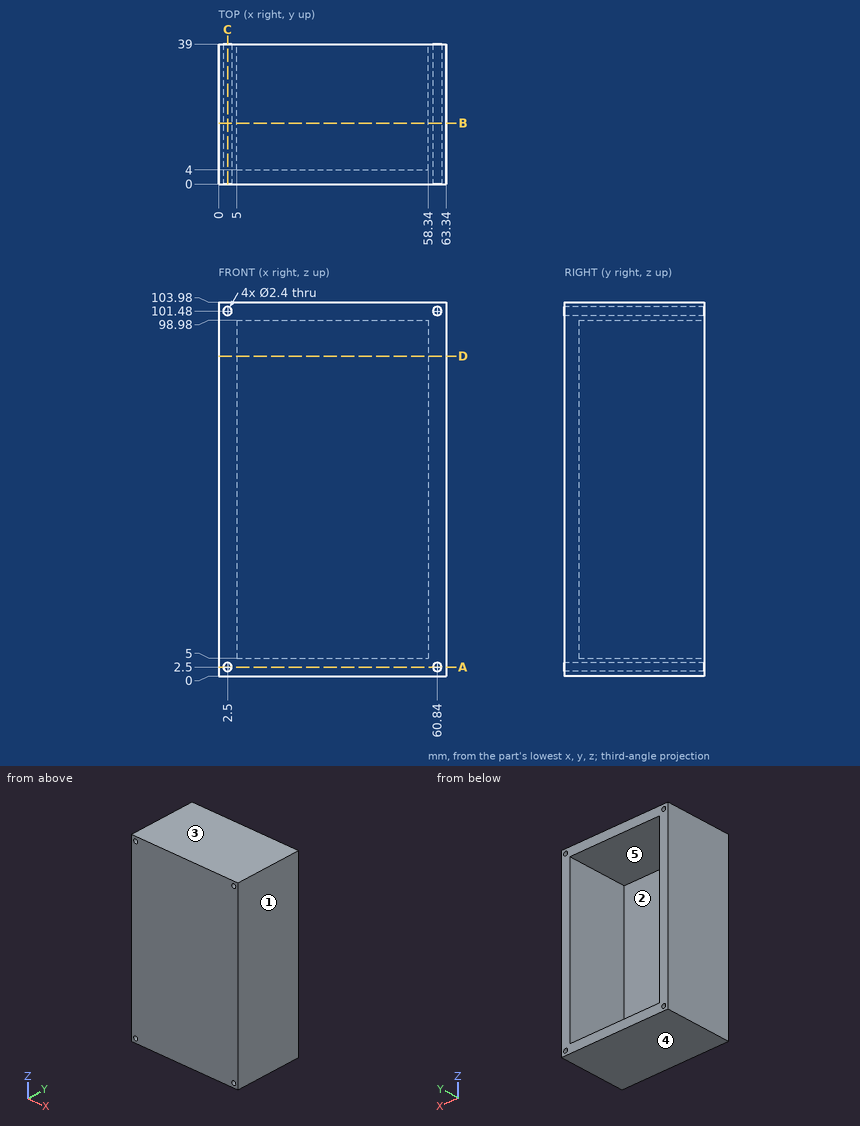
Answer from the drawing. Dimensions are ordinates in mm from the lowest x, y and z of the part. A direction names the side the tool comes from. Round coordinates to 2 decimals unless told otherwise and drop trailing zeros. Write each loop counter-clockwise with the first axis right and the second up, starting at its lowest first coordinate (ties: lowest second). Pieces come first, ordered by that corner, then holes.
1. The part is cut by section C-C, the plane x = 2.5. Determine the outline of the cut face in (y, z).
2. Determine the mould class of the marked faces 1, 2 and 3 for opening direction Z: pulls with the +Z half, pulls with the -Z half, needs draft (parallel to the pull), parting line crosses it, or undercut.
3. The part is cut by section D-D, the plane z = 89. Determine the outline of the cut face in (x, y).
4. Straight lines are drawn through the part: L1, parallel to Z at x = 60.84, y = 22; L2, parallel to X at y = 19, z = 101.48; L3, parallel to X at y = 15, z = 62.5. For each, find the intervals that lie inside material, in ascending order.
5. Which of the six approach directions +Z, -Z, +X, -X, +Y, -Y give full straight-line access (tool end or side, diameter ignored) to the marked faces 4 and 5?
6. Given pin 1 Ø6 at (x, z) = (10, 23.5) entering from -Y; pin 2 Ø10 at (x, z) = (10.5, 82) entering from +Y; pin 3 Ø1.4 at (x, z) = (2.5, 101.48) entering from +Y, each flat-ended and moving along its own axis, determine where each tip first touches the part or whether it passes through.
7. The part is cut by section A-A, the plane z = 2.5. Determine the outline of the cut face in (x, y).
8. The part is cut by section B-B, the plane y = 17. Determine the outline of the cut face in (x, z), then the cut area to 3 significant figures.
Values:
1. outline: (0, 0) - (39, 0) - (39, 1.3) - (0, 1.3) - close; (0, 3.7) - (39, 3.7) - (39, 100.28) - (0, 100.28) - close; (0, 102.68) - (39, 102.68) - (39, 103.98) - (0, 103.98) - close
2. face 1: needs draft
2. face 2: undercut
2. face 3: pulls with the +Z half
3. outline: (0, 0) - (63.34, 0) - (63.34, 39) - (58.34, 39) - (58.34, 4) - (5, 4) - (5, 39) - (0, 39) - close
4. L1: z = 0 to 1.3, 3.7 to 100.28, 102.68 to 103.98
4. L2: x = 0 to 1.3, 3.7 to 59.64, 62.04 to 63.34
4. L3: x = 0 to 5, 58.34 to 63.34
5. face 4: -Z, +X, -X, +Y, -Y
5. face 5: +Y
6. pin 1: stops at y = 0
6. pin 2: stops at y = 4
6. pin 3: passes through
7. outline: (0, 0) - (1.3, 0) - (1.3, 39) - (0, 39) - close; (3.7, 0) - (59.64, 0) - (59.64, 39) - (3.7, 39) - close; (62.04, 0) - (63.34, 0) - (63.34, 39) - (62.04, 39) - close
8. outline: (0, 0) - (63.34, 0) - (63.34, 103.98) - (0, 103.98) - close; hole circle Ø2.4 at (2.5, 2.5); hole circle Ø2.4 at (2.5, 101.48); hole (5, 5) - (58.34, 5) - (58.34, 98.98) - (5, 98.98) - close; hole circle Ø2.4 at (60.84, 2.5); hole circle Ø2.4 at (60.84, 101.48)
8. area: 1,560 mm2
